from build123d import *

# Parameters (mm, degrees)
SKETCH1_R           = 26.590625
BOSS_EXTRUDE1_DEPTH = 1.5875
SKETCH2_R           = 25.5984375
BOSS_EXTRUDE2_DEPTH = 2.38125
SKETCH3_R           = 26.590625
BOSS_EXTRUDE3_DEPTH = 1.5875
SKETCH5_R           = 9.525
BOSS_EXTRUDE4_DEPTH = 0.79375
SKETCH6_R           = 3.96875
CUT_EXTRUDE1_DEPTH  = 39.137188881
FILLET1_R           = 1
FILLET2_R           = 1


with BuildPart() as part:
    # Sketch1 → Boss-Extrude1 (new body)
    with BuildSketch(Plane(origin=(0, 0, 0), x_dir=(1, 0, 0), z_dir=(0, 1, 0))):
        with Locations(Location((0, 0, 0), (0, 0, 270))):
            Circle(SKETCH1_R)
    extrude(amount=BOSS_EXTRUDE1_DEPTH)

    # Sketch2 → Boss-Extrude2 (add)
    with BuildSketch(Plane(origin=(0, 1.5875, 0), x_dir=(1, 0, 0), z_dir=(0, 1, 0))):
        with Locations(Location((0, 0, 0), (0, 0, 90))):
            Circle(SKETCH2_R)
    extrude(amount=BOSS_EXTRUDE2_DEPTH)

    # Sketch3 → Boss-Extrude3 (add)
    with BuildSketch(Plane(origin=(0, 3.96875, 0), x_dir=(1, 0, 0), z_dir=(0, 1, 0))):
        with Locations(Location((0, 0, 0), (0, 0, 270))):
            Circle(SKETCH3_R)
    extrude(amount=BOSS_EXTRUDE3_DEPTH)

    # Sketch5 → Boss-Extrude4 (add)
    with BuildSketch(Plane(origin=(0, 5.55625, 0), x_dir=(1, 0, 0), z_dir=(0, 1, 0))):
        with Locations(Location((0, 0, 0), (0, 0, 270))):
            Circle(SKETCH5_R)
    extrude(amount=BOSS_EXTRUDE4_DEPTH)

    # Sketch6 → Cut-Extrude1 (cut, through all)
    with BuildSketch(Plane(origin=(0, 6.35, 0), x_dir=(1, 0, 0), z_dir=(0, 1, 0))):
        with Locations(Location((0, 0, 0), (0, 0, 270))):
            Circle(SKETCH6_R)
    extrude(amount=-CUT_EXTRUDE1_DEPTH, mode=Mode.SUBTRACT)

    # Fillet1
    # the kernel refuses this fillet: 1 mm, written as the material it adds along each edge
    with BuildSketch(Plane(origin=(0, 1.5875, 0), x_dir=(0, 0, -1), z_dir=(1, 0, 0))) as fillet1_piece_1_section:
        with BuildLine():
            CenterArc((25.5984375 + FILLET1_R, FILLET1_R), FILLET1_R, 180, 90)
            Line((25.5984375 + FILLET1_R, 0), (25.5984375, 0))
            Line((25.5984375, 0), (25.5984375, FILLET1_R))
        make_face()
    fillet1_piece_1 = revolve(axis=Axis((0, 1.5875, 0), (0, 1, 0)), mode=Mode.PRIVATE)
    fillet1_piece_1 = fillet1_piece_1 & Plane(origin=(0, 1.858804506, 0), x_dir=(0, 0, 1), z_dir=(0, -1, 0)) * Cylinder(26.590625, 107, mode=Mode.PRIVATE)
    add(fillet1_piece_1)

    # Fillet2
    # the kernel refuses this fillet: 1 mm, written as the material it adds along each edge
    with BuildSketch(Plane(origin=(0, 3.96875, 0), x_dir=(0, 0, -1), z_dir=(1, 0, 0))) as fillet2_piece_1_section:
        with BuildLine():
            CenterArc((25.5984375 + FILLET2_R, -FILLET2_R), FILLET2_R, 90, 90)
            Line((25.5984375 + FILLET2_R, 0), (25.5984375, 0))
            Line((25.5984375, 0), (25.5984375, -FILLET2_R))
        make_face()
    fillet2_piece_1 = revolve(axis=Axis((0, 3.96875, 0), (0, 1, 0)), mode=Mode.PRIVATE)
    fillet2_piece_1 = fillet2_piece_1 & Plane(origin=(0, 3.697445494, 0), x_dir=(0, 0, 1), z_dir=(0, -1, 0)) * Cylinder(26.590625, 107, mode=Mode.PRIVATE)
    add(fillet2_piece_1)


solid = part.part
CAD build for the part. Positions are in the model's coordinates, mm. A direction names the side the tool comes from. Give positions to 0.01 mm unless a question says otherwise; leave off trailing zeros. Loops run counter-clockwise (first coordinate to the right, second up) from the corner with the lowest first, then second, coordinate; pieces in that order, holes last. Notation, with made-up numbers: M 45.25,21.25 L 93.25,21.25 A15 cw 93.25,40.25 Z; hole C 70,60.25 d5. An arc over 180 degrees is marked long. Write each question's results on one line, items separated by ' | '.
Q1. Band-saw the part on C-C on y = 4.75. Write the cut outline in (x, z), and give its area (3 significant figures).
Geometry check:
outline: C 0,0 d53.18; hole C 0,0 d7.94 | area: 2,170 mm²
Q2. Which spindle directions (+Z, -Z, +X, -X, +Y, -Y) get a long thin tool onto all of the face, cutting with end or side? Do faces 1 (the face through (10.184, 4.751, 24.563)), 2 (the face through (22.71, 2.78, -11.81)), 3 (the face through (-11, 5.556, 0)). Say none if no direction does.
Geometry check:
face 1: +Y, -Y | face 2: none | face 3: +Y
Q3. Probe probe 1 along X at (y, z) = (3, 0); probe 2 along X at (y, z) = (4.5, 0); probe 3 along Y at (x, z) = (-20.5, 10). List the from-to ranges inside material, lowest first.
Geometry check:
probe 1: x = -25.6 to -3.97, 3.97 to 25.6 | probe 2: x = -26.59 to -3.97, 3.97 to 26.59 | probe 3: y = 0 to 5.56
Q4. Flat gauge pins, fed straight in: P1, Ø8, axis at x = 7, z = -1.5, coming from the -Y side; P2, Ø5, axis at x = -11, z = -11, coming from the +Y side; P3, Ø7, axis at x = 0, z = 0, coming from the +Y side. Where does each tip first touch, or does it go through?
Geometry check:
P1: stops at y = 0 | P2: stops at y = 5.56 | P3: passes through
Q5. Mould opens along Z. For faces 4 (the face through (-4, 6.35, 2)), 5 (the face through (-3.874, 3.219, -0.86)), 6 (the face through (-5.796, 5.948, -7.559)) say: pulls with the +Z half, pulls with the -Z half, needs draft (parallel to the pull), parting line crosses it, or undercut.
Geometry check:
face 4: needs draft | face 5: undercut | face 6: parting line crosses it
